```python
from build123d import *

# Parameters (mm, degrees)
SZKIC1_W                    = 75
SZKIC1_H                    = 75
DODANIE_WYCI_GNI_CIE1_DEPTH = 10
ZAOKR_GLENIE1_R             = 5
WYTNIJ_WYCI_GNI_CIE1_DEPTH  = 8
WYTNIJ_WYCI_GNI_CIE2_DEPTH  = 4
SZKIC7_R                    = 1.9
SZKIC7_R_2                  = 0.9
SZKIC7_R_3                  = 1.900523095
SZKIC7_R_4                  = 0.900523095
DODANIE_WYCI_GNI_CIE2_DEPTH = 8.7
SZKIC9_R                    = 0.900523095
SZKIC9_R_2                  = 0.9
DODANIE_WYCI_GNI_CIE3_DEPTH = 1
SZKIC10_R                   = 1.25
DODANIE_WYCI_GNI_CIE4_DEPTH = 1
SZKIC11_R                   = 2
SZKIC11_R_2                 = 1.25
DODANIE_WYCI_GNI_CIE5_DEPTH = 8.5
WYTNIJ_WYCI_GNI_CIE20_DEPTH = 10
SZKIC22_W                   = 4
SZKIC22_H                   = 1
DODANIE_WYCI_GNI_CIE6_DEPTH = 0.3
SZKIC24_W                   = 4
SZKIC24_H                   = 1
DODANIE_WYCI_GNI_CIE7_DEPTH = 0.3
WYTNIJ_WYCI_GNI_CIE13_DEPTH = 55
WYTNIJ_WYCI_GNI_CIE14_DEPTH = 55


with BuildPart() as part:
    # Szkic1 → Dodanie-wyciągnięcie1 (new body)
    with BuildSketch(Plane(origin=(0, 0, 0), x_dir=(1, 0, 0), z_dir=(0, 1, 0))):
        with Locations((37.5, 37.5)):
            Rectangle(SZKIC1_W, SZKIC1_H)
    extrude(amount=DODANIE_WYCI_GNI_CIE1_DEPTH)

    # Zaokrąglenie1
    zaokr_glenie1_edges = [part.edges().sort_by_distance(p)[0] for p in [
        (0, 5, 0),
        (0, 5, -75),
        (75, 5, -75),
        (75, 5, 0),
    ]]
    fillet(zaokr_glenie1_edges, radius=ZAOKR_GLENIE1_R)

    # Szkic4 → Wytnij-wyciągnięcie1 (cut)
    with BuildSketch(Plane(origin=(0, 10, 0), x_dir=(1, 0, 0), z_dir=(0, 1, 0))):
        with BuildLine():
            Line((2, 70), (2, 5))
            ThreePointArc((2, 5), (2.878679656, 2.878679656), (5, 2))
            Line((5, 2), (70, 2))
            ThreePointArc((70, 2), (72.121320344, 2.878679656), (73, 5))
            Line((73, 5), (73, 70))
            ThreePointArc((73, 70), (72.121320344, 72.121320344), (70, 73))
            Line((70, 73), (5, 73))
            ThreePointArc((5, 73), (2.878679656, 72.121320344), (2, 70))
        make_face()
    extrude(amount=-WYTNIJ_WYCI_GNI_CIE1_DEPTH, mode=Mode.SUBTRACT)

    # Szkic6 → Wytnij-wyciągnięcie2 (cut)
    with BuildSketch(Plane(origin=(0, 10, 0), x_dir=(1, 0, 0), z_dir=(0, 1, 0))):
        with BuildLine():
            Line((1, 70), (1, 5))
            ThreePointArc((1, 5), (2.171572875, 2.171572875), (5, 1))
            Line((5, 1), (70, 1))
            ThreePointArc((70, 1), (72.828427125, 2.171572875), (74, 5))
            Line((74, 5), (74, 70))
            ThreePointArc((74, 70), (72.828427125, 72.828427125), (70, 74))
            Line((70, 74), (5, 74))
            ThreePointArc((5, 74), (2.171572875, 72.828427125), (1, 70))
        make_face()
        with BuildLine():
            Line((2, 70), (2, 5))
            ThreePointArc((2, 5), (2.878679656, 2.878679656), (5, 2))
            Line((5, 2), (70, 2))
            ThreePointArc((70, 2), (72.121320344, 2.878679656), (73, 5))
            Line((73, 5), (73, 70))
            ThreePointArc((73, 70), (72.121320344, 72.121320344), (70, 73))
            Line((70, 73), (5, 73))
            ThreePointArc((5, 73), (2.878679656, 72.121320344), (2, 70))
        make_face(mode=Mode.SUBTRACT)
    extrude(amount=-WYTNIJ_WYCI_GNI_CIE2_DEPTH, mode=Mode.SUBTRACT)

    # Szkic7 → Dodanie-wyciągnięcie2 (add)
    # profile 1 of 4: a face of its own
    with BuildSketch(Plane(origin=(0, 2, 0), x_dir=(1, 0, 0), z_dir=(0, 1, 0))):
        with Locations(Location((24, 52, 0), (0, 0, 270))):
            Circle(SZKIC7_R)
        with Locations(Location((24, 52, 0), (0, 0, 270))):
            Circle(SZKIC7_R_2, mode=Mode.SUBTRACT)
    # profile 2 of 4: a face of its own
    with BuildSketch(Plane(origin=(0, 2, 0), x_dir=(1, 0, 0), z_dir=(0, 1, 0))):
        with Locations(Location((35.5, 52, 0), (0, 0, 270))):
            Circle(SZKIC7_R_3)
        with Locations(Location((35.5, 52, 0), (0, 0, 270))):
            Circle(SZKIC7_R_4, mode=Mode.SUBTRACT)
    # profile 3 of 4: a face of its own
    with BuildSketch(Plane(origin=(0, 2, 0), x_dir=(1, 0, 0), z_dir=(0, 1, 0))):
        with Locations(Location((35.5, 5, 0), (0, 0, 270))):
            Circle(SZKIC7_R)
        with Locations(Location((35.5, 5, 0), (0, 0, 270))):
            Circle(SZKIC7_R_2, mode=Mode.SUBTRACT)
    # profile 4 of 4: a face of its own
    with BuildSketch(Plane(origin=(0, 2, 0), x_dir=(1, 0, 0), z_dir=(0, 1, 0))):
        with Locations(Location((24, 5, 0), (0, 0, 270))):
            Circle(SZKIC7_R)
        with Locations(Location((24, 5, 0), (0, 0, 270))):
            Circle(SZKIC7_R_2, mode=Mode.SUBTRACT)
    extrude(amount=DODANIE_WYCI_GNI_CIE2_DEPTH)

    # Szkic9 → Dodanie-wyciągnięcie3 (add)
    with BuildSketch(Plane(origin=(0, 2, 0), x_dir=(1, 0, 0), z_dir=(0, 1, 0))):
        with Locations(Location((35.5, 52, 0), (0, 0, 270))):
            Circle(SZKIC9_R)
        with Locations(Location((35.5, 5, 0), (0, 0, 270))):
            Circle(SZKIC9_R_2)
        with Locations(Location((24, 5, 0), (0, 0, 270))):
            Circle(SZKIC9_R_2)
        with Locations(Location((24, 52, 0), (0, 0, 270))):
            Circle(SZKIC9_R_2)
    extrude(amount=DODANIE_WYCI_GNI_CIE3_DEPTH)

    # Szkic10 → Dodanie-wyciągnięcie4 (add)
    with BuildSketch(Plane(origin=(0, 2, 0), x_dir=(1, 0, 0), z_dir=(0, 1, 0))):
        with Locations(Location((67, 23.5, 0), (0, 0, 270))):
            Circle(SZKIC10_R)
        with Locations(Location((67, 8, 0), (0, 0, 270))):
            Circle(SZKIC10_R)
    extrude(amount=DODANIE_WYCI_GNI_CIE4_DEPTH)

    # Szkic11 → Dodanie-wyciągnięcie5 (add)
    # profile 1 of 2: a face of its own
    with BuildSketch(Plane(origin=(0, 2, 0), x_dir=(1, 0, 0), z_dir=(0, 1, 0))):
        with Locations(Location((67, 23.5, 0), (0, 0, 270))):
            Circle(SZKIC11_R)
        with Locations(Location((67, 23.5, 0), (0, 0, 270))):
            Circle(SZKIC11_R_2, mode=Mode.SUBTRACT)
    # profile 2 of 2: a face of its own
    with BuildSketch(Plane(origin=(0, 2, 0), x_dir=(1, 0, 0), z_dir=(0, 1, 0))):
        with Locations(Location((67, 8, 0), (0, 0, 270))):
            Circle(SZKIC11_R)
        with Locations(Location((67, 8, 0), (0, 0, 270))):
            Circle(SZKIC11_R_2, mode=Mode.SUBTRACT)
    extrude(amount=DODANIE_WYCI_GNI_CIE5_DEPTH)

    # Szkic19 → Wytnij-wyciągnięcie20 (cut)
    with BuildSketch(Plane(origin=(0, 0, -2), x_dir=(-1, 0, 0), z_dir=(0, 0, -1))):
        Polygon((-34.25, 10), (-25.25, 10), (-25.25, 8.5), (-26.5, 8.5), (-32.5, 8.5), (-34.25, 8.5), align=None)
    extrude(amount=-WYTNIJ_WYCI_GNI_CIE20_DEPTH, mode=Mode.SUBTRACT)

    # Szkic22 → Dodanie-wyciągnięcie6 (add)
    with BuildSketch(Plane.ZY.offset(-74)):
        with Locations((-37.5, 9.5)):
            Rectangle(SZKIC22_W, SZKIC22_H)
        with Locations((-63, 9.5)):
            Rectangle(SZKIC22_W, SZKIC22_H)
        with Locations((-12, 9.5)):
            Rectangle(SZKIC22_W, SZKIC22_H)
    extrude(amount=DODANIE_WYCI_GNI_CIE6_DEPTH)

    # Szkic24 → Dodanie-wyciągnięcie7 (add)
    with BuildSketch(Plane(origin=(1, 0, 0), x_dir=(0, 0, -1), z_dir=(1, 0, 0))):
        with Locations((12, 9.5)):
            Rectangle(SZKIC24_W, SZKIC24_H)
        with Locations((63, 9.5)):
            Rectangle(SZKIC24_W, SZKIC24_H)
        with Locations((37.5, 9.5)):
            Rectangle(SZKIC24_W, SZKIC24_H)
    extrude(amount=DODANIE_WYCI_GNI_CIE7_DEPTH)

    # Szkic25 → Wytnij-wyciągnięcie13 (cut)
    with BuildSketch(Plane.XY.offset(-10)):
        Polygon((1, 10), (1.3, 9.5), (1.3, 10), align=None)
    extrude(amount=-WYTNIJ_WYCI_GNI_CIE13_DEPTH, mode=Mode.SUBTRACT)

    # Szkic26 → Wytnij-wyciągnięcie14 (cut)
    with BuildSketch(Plane(origin=(0, 0, -65), x_dir=(-1, 0, 0), z_dir=(0, 0, -1))):
        Polygon((-74, 10), (-73.7, 10), (-73.7, 9.5), align=None)
    extrude(amount=-WYTNIJ_WYCI_GNI_CIE14_DEPTH, mode=Mode.SUBTRACT)


with BuildPart() as body_2:
    # Lustro5: mirrored copy
    add(part.part.mirror(Plane.ZX.offset(-10)))


solid = body_2.part
```
Can you work these out from the model? Positions are in its coordinate system, mm. Coordinates: 2 decimals unless noted, no trailing zeros. Loops run counter-clockwise (first coordinate to the right, second up) from the corner with the lowest first, then second, coordinate; pieces in that order, holes last. Notation, with made-up numbers: (83, -20.5) - (142, -20.5) arc R35 cw to (142, 16.5) - close; hole circle Ø8 at (21, -21.75). An arc over 180 degrees is marked (long way). Use a Markdown table: item, result.
Item 1: Will these pins go through, and if not, where does the flat tip stop? pin 1 (0.9 mm diameter, centred on x = 24, z = -52.5, fed in from -Y); pin 2 (1.2 mm diameter, centred on x = 67, z = -7.5, fed in from -Y); pin 3 (10 mm diameter, centred on x = 11.5, z = -52, fed in from -Y).
Numbers:
| item | result |
|---|---|
| pin 1 | stops at y = -30.7 |
| pin 2 | stops at y = -23 |
| pin 3 | stops at y = -22 |
Item 2: I want a section at B-B on z = -52. Please give me the cut outline in (x, y), and give its area (3 significant figures).
Numbers:
| item | result |
|---|---|
| outline | (0, -30) - (1, -30) - (1, -26) - (2, -26) - (2, -22) - (22.1, -22) - (22.1, -30.7) - (23.1, -30.7) - (23.1, -23) - (24.9, -23) - (24.9, -30.7) - (25.9, -30.7) - (25.9, -22) - (33.6, -22) - (33.6, -30.7) - (34.6, -30.7) - (34.6, -23) - (36.4, -23) - (36.4, -30.7) - (37.4, -30.7) - (37.4, -22) - (73, -22) - (73, -26) - (74, -26) - (74, -30) - (75, -30) - (75, -20) - (0, -20) - close |
| area | 212 mm2 |
Item 3: We'd pull the mould along X, two halves only. Please class faces 1 (the face through (36.39, -26.8, -5.12)), 2 (the face through (37, -25, 0)), 3 (the face through (0, -25, -37)): released by +X, released by -X, zero draft, split by the parting line, or undercut.
Numbers:
| item | result |
|---|---|
| face 1 | undercut |
| face 2 | zero draft |
| face 3 | released by -X |
Item 4: I want a section at D-D on z = -23.5. Please give me the cut outline in (x, y).
Numbers:
| item | result |
|---|---|
| outline | (0, -30) - (1, -30) - (1, -26) - (2, -26) - (2, -22) - (65, -22) - (65, -30.5) - (65.75, -30.5) - (65.75, -23) - (68.25, -23) - (68.25, -30.5) - (69, -30.5) - (69, -22) - (73, -22) - (73, -26) - (74, -26) - (74, -30) - (75, -30) - (75, -20) - (0, -20) - close |
Item 5: I want a section at C-C on x = 24. Please give me the cut outline in (y, z).
Numbers:
| item | result |
|---|---|
| outline | (-30.7, -53.9) - (-22, -53.9) - (-22, -73) - (-26, -73) - (-26, -74) - (-30, -74) - (-30, -75) - (-20, -75) - (-20, 0) - (-30, 0) - (-30, -1) - (-26, -1) - (-26, -2) - (-22, -2) - (-22, -3.1) - (-30.7, -3.1) - (-30.7, -4.1) - (-23, -4.1) - (-23, -5.9) - (-30.7, -5.9) - (-30.7, -6.9) - (-22, -6.9) - (-22, -50.1) - (-30.7, -50.1) - (-30.7, -51.1) - (-23, -51.1) - (-23, -52.9) - (-30.7, -52.9) - close |
Item 6: I want a section at A-A on x = 16. Please give me the cut outline in (y, z).
Numbers:
| item | result |
|---|---|
| outline | (-30, -75) - (-20, -75) - (-20, 0) - (-30, 0) - (-30, -1) - (-26, -1) - (-26, -2) - (-22, -2) - (-22, -73) - (-26, -73) - (-26, -74) - (-30, -74) - close |
Item 7: If I drill on probe 1 along X at (y, z) = (-28.5, -52); probe 2 along X at (y, z) = (-27, -8); probe 3 along X at (y, z) = (-25.5, -23.5), over which ranges is the centre line in solid material (lowest first)? Write a range as from..to.
Numbers:
| item | result |
|---|---|
| probe 1 | x = 0..1, 22.1..23.1, 24.9..25.9, 33.6..34.6, 36.4..37.4, 74..75 |
| probe 2 | x = 0..1, 65..65.75, 68.25..69, 74..75 |
| probe 3 | x = 0..2, 65..65.75, 68.25..69, 73..75 |
